```python
from build123d import *

# Parameters (mm, degrees)
SKETCH009_R             = 17.5
PAD008_DEPTH            = 11.5
CHAMFER_1_SIZE2         = 0.25
CHAMFER_1_SIZE          = 1.5
CHAMFER_2_SIZE2         = 0.25
CHAMFER_2_SIZE          = 1.5
CHAMFER_3_SIZE2         = 0.25
CHAMFER_3_SIZE          = 1.5
CHAMFER_4_SIZE2         = 0.25
CHAMFER_4_SIZE          = 1.5
SKETCH016_R             = 17.5
PAD012_DEPTH            = 3
CHAMFER003_1_SIZE2      = 0.25
CHAMFER003_1_SIZE       = 1.5
CHAMFER003_2_SIZE2      = 0.25
CHAMFER003_2_SIZE       = 1.5
SKETCH017_R             = 17.5
SKETCH017_R_2           = 13.75
PAD013_DEPTH            = 1
BODY001_PLACEMENT_ANGLE = 180


with BuildPart() as part:
    # Sketch009 → Pad008 (new body)
    with BuildSketch(Plane.XY.offset(20.75)):
        Circle(SKETCH009_R)
        with BuildLine():
            Line((-8.346636, 11.856798), (-8.000833, 11.257849))
            Line((-8.000833, 11.257849), (-5.749167, 12.557849))
            Line((-5.749167, 12.557849), (-6.09497, 13.156798))
            ThreePointArc((14.387842, 1.8), (7.031155, 12.681201), (-6.09497, 13.156798))
            Line((14.387842, 1.8), (13.75, 1.8))
            Line((13.75, 1.8), (13.75, -1.8))
            Line((14.387842, -1.8), (13.75, -1.8))
            ThreePointArc((-6.09497, -13.156798), (7.031155, -12.681201), (14.387842, -1.8))
            Line((-5.749167, -12.557849), (-6.09497, -13.156798))
            Line((-8.000833, -11.257849), (-5.749167, -12.557849))
            Line((-8.346636, -11.856798), (-8.000833, -11.257849))
            ThreePointArc((-8.346636, 11.856798), (-14.5, 0), (-8.346636, -11.856798))
        make_face(mode=Mode.SUBTRACT)
    extrude(amount=-PAD008_DEPTH)

    # Chamfer 1
    chamfer_1_edges = [part.edges().sort_by_distance(p)[0] for p in [
        (-8.173735, -11.557324, 9.25),
    ]]
    chamfer_1_side = part.faces().sort_by_distance((-8.173735, -11.557324, 15))[0]
    chamfer(chamfer_1_edges, length=CHAMFER_1_SIZE, length2=CHAMFER_1_SIZE2, reference=chamfer_1_side)

    # Chamfer 2
    chamfer_2_edges = [part.edges().sort_by_distance(p)[0] for p in [
        (-5.922069, -12.857324, 9.25),
    ]]
    chamfer_2_side = part.faces().sort_by_distance((-5.922069, -12.857324, 15))[0]
    chamfer(chamfer_2_edges, length=CHAMFER_2_SIZE, length2=CHAMFER_2_SIZE2, reference=chamfer_2_side)

    # Chamfer 3
    chamfer_3_edges = [part.edges().sort_by_distance(p)[0] for p in [
        (-8.173735, 11.557324, 9.25),
    ]]
    chamfer_3_side = part.faces().sort_by_distance((-8.173735, 11.557324, 15))[0]
    chamfer(chamfer_3_edges, length=CHAMFER_3_SIZE, length2=CHAMFER_3_SIZE2, reference=chamfer_3_side)

    # Chamfer 4
    chamfer_4_edges = [part.edges().sort_by_distance(p)[0] for p in [
        (-5.922069, 12.857324, 9.25),
    ]]
    chamfer_4_side = part.faces().sort_by_distance((-5.922069, 12.857324, 15))[0]
    chamfer(chamfer_4_edges, length=CHAMFER_4_SIZE, length2=CHAMFER_4_SIZE2, reference=chamfer_4_side)

    # Sketch016 → Pad012 (join)
    with BuildSketch(Plane.XY.offset(9.25)):
        Circle(SKETCH016_R)
        with BuildLine():
            Line((14.387842, 1.8), (13.75, 1.8))
            Line((13.75, 1.8), (13.75, -1.8))
            Line((14.387842, -1.8), (13.75, -1.8))
            ThreePointArc((14.387842, 1.8), (-14.5, 0), (14.387842, -1.8))
        make_face(mode=Mode.SUBTRACT)
    extrude(amount=-PAD012_DEPTH)

    # Chamfer003 1
    chamfer003_1_edges = [part.edges().sort_by_distance(p)[0] for p in [
        (14.068921, -1.8, 6.25),
    ]]
    chamfer003_1_side = part.faces().sort_by_distance((14.068921, -1.8, 7.75))[0]
    chamfer(chamfer003_1_edges, length=CHAMFER003_1_SIZE, length2=CHAMFER003_1_SIZE2, reference=chamfer003_1_side)

    # Chamfer003 2
    chamfer003_2_edges = [part.edges().sort_by_distance(p)[0] for p in [
        (14.068921, 1.8, 6.25),
    ]]
    chamfer003_2_side = part.faces().sort_by_distance((14.068921, 1.8, 7.75))[0]
    chamfer(chamfer003_2_edges, length=CHAMFER003_2_SIZE, length2=CHAMFER003_2_SIZE2, reference=chamfer003_2_side)

    # Sketch017 → Pad013 (join)
    with BuildSketch(Plane.XY.offset(20.75)):
        Circle(SKETCH017_R)
        Circle(SKETCH017_R_2, mode=Mode.SUBTRACT)
    extrude(amount=PAD013_DEPTH)


with BuildPart() as part_1:
    # Body001 placement: moved
    add(part.part.moved(Location((0, 0, 0.13))).rotate(Axis((0, 0, 0.13), (0, 0, 1)), BODY001_PLACEMENT_ANGLE))


solid = part_1.part
```
Work out the finished part from the listing and answer in its coordinate system (mm). A direction names the side the tool comes from. Coordinates: 2 decimals unless noted, no trailing zeros. Write each loop counter-clockwise with the first axis right and the second up, starting at its lowest first coordinate (ties: lowest second). Pieces come first, ordered by that corner, then holes. Notation, with made-up numbers: (37, 16.25) - (66, 16.25) arc R4 cw to (66, 23.25) - close; hole circle Ø1 at (69, 27.5). An arc over 180 degrees is marked (long way). Answer as a JSON object with one key per item and string values.
Q1. Consider L1, parallel to Y at x = 0, z = 7.4; L2, parallel to X at y = 0.5, z = 14.5; L3, parallel to Y at x = -4, z = 14.5. Determine where each line is inside the solid, lowest interval first. Write a range as from..to.
Results list:
{"L1": "y = -17.5..-14.5, 14.5..17.5", "L2": "x = -17.49..-13.75, 14.49..17.49", "L3": "y = -17.04..-13.94, 13.94..17.04"}
Q2. Find section A-A (x = 0). Write down the section's boundary in (y, z), plus the area to 3 significant figures.
Results list:
{"outline": "(-17.5, 6.38) - (-14.5, 6.38) - (-14.5, 20.88) - (-13.75, 20.88) - (-13.75, 21.88) - (-17.5, 21.88) - close; (13.75, 20.88) - (14.5, 20.88) - (14.5, 6.38) - (17.5, 6.38) - (17.5, 21.88) - (13.75, 21.88) - close", "area": "94.5 mm^2"}
Q3. Given pin 1 Ø0.8 at (x, y) = (6.5, 12) entering from -Z; pin 2 Ø5 at (x, z) = (-3.5, 19.5) entering from -Y; pin 3 Ø0.5 at (x, z) = (-14, 15.5) entering from -Y; pin 4 Ø3 at (x, y) = (11, -0.5) entering from +Z, each flat-ended and moving along its own axis, determine where each tip first touches the part or whether it passes through.
Results list:
{"pin 1": "stops at z = 9.38", "pin 2": "stops at y = -17.47", "pin 3": "stops at y = -10.83", "pin 4": "passes through"}
Q4. Find section C-C (y = 7). Write down the section's boundary in (x, z).
Results list:
{"outline": "(-16.04, 6.38) - (-12.7, 6.38) - (-12.7, 20.88) - (-11.83, 20.88) - (-11.83, 21.88) - (-16.04, 21.88) - close; (11.83, 20.88) - (12.7, 20.88) - (12.7, 6.38) - (16.04, 6.38) - (16.04, 21.88) - (11.83, 21.88) - close"}
Q5. Find section D-D (x = 15). Write down the section's boundary in (y, z), plus the area to 3 significant figures.
Results list:
{"outline": "(-9.01, 6.38) - (9.01, 6.38) - (9.01, 21.88) - (-9.01, 21.88) - close", "area": "279 mm^2"}
Q6. Find section B-B (z = 18.5). Write down the section's boundary in (x, y).
Results list:
{"outline": "circle Ø35 at (0, 0); hole (-14.39, -1.8) arc R14.5 ccw to (6.09, -13.16) - (5.75, -12.56) - (8, -11.26) - (8.35, -11.86) arc R14.5 ccw to (8.35, 11.86) - (8, 11.26) - (5.75, 12.56) - (6.09, 13.16) arc R14.5 ccw to (-14.39, 1.8) - (-13.75, 1.8) - (-13.75, -1.8) - close"}
Q7. For a pull along X with two mould halves and no side action, classify faces 3 (the flat face through (4, 14.2, 6.38)), 4 (the cylindrical face through (3.794, 17.084, 14.022)), 5 (the flat face through (-6, 13, 20.88)) as pulls with the +X half, pulls with the -X half, needs draft (parallel to the pull), parting line crosses it, or undercut.
Results list:
{"face 3": "needs draft", "face 4": "parting line crosses it", "face 5": "undercut"}
Q8. Which of the six approach directions +Z, -Z, +X, -X, +Y, -Y give full straight-line access (tool end or side, diameter ignored) to faces 1 (the flat face through (-8, 12, 21.88)), 2 (the flat face through (6.89, 11.9, 15.21))?
Results list:
{"face 1": "+Z, +X, -X, +Y, -Y", "face 2": "-Z"}
